from build123d import *

# Parameters (mm, degrees)
ESQUISSE2_R                = 7
ESQUISSE2_R_2              = 4
ESQUISSE2_R_3              = 23
BASE_EXTRUSION_DEPTH       = 2.5
ESQUISSE9_R                = 1.7
ENL_V_MAT_EXTRU_2_DEPTH    = 146.323213238
R_P_TITION_LIN_AIRE1_COUNT = 2
R_P_TITION_LIN_AIRE1_PITCH = 10
ESQUISSE10_R               = 1.7
ENL_V_MAT_EXTRU_3_DEPTH    = 146.323213238
R_P_TITION_LIN_AIRE2_COUNT = 2
R_P_TITION_LIN_AIRE2_PITCH = 83.5


with BuildPart() as part:
    # Esquisse2 → Base-Extrusion (new body)
    with BuildSketch(Plane.XY):
        with BuildLine():
            Line((-60.587831126, 50.043046358), (101.412168874, 50.043046358))
            ThreePointArc((101.412168874, 50.043046358), (136.412168874, 15.043046358), (101.412168874, -19.956953642))
            Line((101.412168874, -19.956953642), (-60.587831126, -19.956953642))
            ThreePointArc((-60.587831126, -19.956953642), (-95.587831126, 15.043046358), (-60.587831126, 50.043046358))
        make_face()
        with Locations((-60.587831126, 15.043046358)):
            Circle(ESQUISSE2_R, mode=Mode.SUBTRACT)
        with Locations((101.412168874, 15.043046358)):
            Circle(ESQUISSE2_R_2, mode=Mode.SUBTRACT)
        with Locations((51.412168874, 15.043046358)):
            Circle(ESQUISSE2_R_3, mode=Mode.SUBTRACT)
        with Locations((-10.587831126, 15.043046358)):
            Circle(ESQUISSE2_R_3, mode=Mode.SUBTRACT)
    extrude(amount=BASE_EXTRUSION_DEPTH)

    # Esquisse9 → Enlèv. mat.-Extru.2 (cut, through all)
    with BuildSketch(Plane.XY.offset(2.5)):
        with Locations((12.412168874, 37.043046358)):
            Circle(ESQUISSE9_R)
    enl_v_mat_extru_2 = extrude(amount=-ENL_V_MAT_EXTRU_2_DEPTH, mode=Mode.SUBTRACT)

    # Répétition linéaire1: Enlèv. mat.-Extru.2 ×2
    with Locations(*[(i * R_P_TITION_LIN_AIRE1_PITCH, 0, 0) for i in range(1, R_P_TITION_LIN_AIRE1_COUNT)]):
        add(enl_v_mat_extru_2, mode=Mode.SUBTRACT)

    # Esquisse10 → Enlèv. mat.-Extru.3 (cut, through all)
    with BuildSketch(Plane.XY.offset(2.5)):
        with Locations((-27.087831126, -13.956953642)):
            Circle(ESQUISSE10_R)
    enl_v_mat_extru_3 = extrude(amount=-ENL_V_MAT_EXTRU_3_DEPTH, mode=Mode.SUBTRACT)

    # Répétition linéaire2: Enlèv. mat.-Extru.3 ×2
    with Locations(*[(i * R_P_TITION_LIN_AIRE2_PITCH, 0, 0) for i in range(1, R_P_TITION_LIN_AIRE2_COUNT)]):
        add(enl_v_mat_extru_3, mode=Mode.SUBTRACT)


solid = part.part
Check sheet for the modelled part. Datum: model origin and axes. Units: mm. Round coordinates to 2 decimals unless told otherwise and drop trailing zeros. Loops run counter-clockwise (first coordinate to the right, second up) from the corner with the lowest first, then second, coordinate; pieces in that order, holes last. Notation, with made-up numbers: M 52,-2.75 L 71,-2.75 A24 cw 71,26.25 Z; hole C -7.75,47 d3. An arc over 180 degrees is marked long. One line per question, with ' | ' between items. Start each with the question number.
Item 1: Section check D-D (x = 35.5). Record the boundary of the cut face in (y, z), and give its area (3 significant figures).
Item 2: Section check C-C (z = 1.1). State how many separate pieces and enclosed holes the cut face has, and give its area (3 significant figures).
Item 3: Scan lines: probe 1 along X at (y, z) = (14, 0.85); probe 2 along X at (y, z) = (14.5, 1.05); probe 3 along Y at (x, z) = (51, 0.15). Record each from-to range of solid material in increasing order.
Item 4: Gauge pin test, flat ends, axial feed: pin 1 Ø5.5 at (x, y) = (56.41, -13.96) entering from -Z; pin 2 Ø7 at (x, y) = (101.41, 15.04) entering from +Z. Record the tip position at first contact, or that the pin passes through.
Item 5: Section check B-B (y = -6). Record the boundary of the cut face in (x, z), and give its area (3 significant figures).
Item 6: Section check A-A (x = 3.5). Record the boundary of the cut face in (y, z), and give its area (3 significant figures).
Item 7: Release check for a two-part mould opening along Y. For faces 1 (the face through (22, 16, 0)), 2 (the face through (-28.84, 1.05, 1.23)), 3 (the face through (136.404, 15.813, 1.232)), 4 (the face through (-65.75, 19.77, 1.23)) record: released by +Y, released by -Y, zero draft, split by the parting line, or undercut.
Worked out:
1) outline: M -19.96,0 L -1.56,0 L -1.56,2.5 L -19.96,2.5 Z; M 31.65,0 L 50.04,0 L 50.04,2.5 L 31.65,2.5 Z | area: 92.0 mm^2
2) separate pieces: 1 | enclosed holes: 8 | area: 11,600 mm^2
3) probe 1: -95.57 to -67.51, -53.67 to -33.56, 12.39 to 28.44, 74.39 to 97.55, 105.27 to 136.4 | probe 2: -95.58 to -67.57, -53.61 to -33.58, 12.41 to 28.42, 74.41 to 97.45, 105.38 to 136.41 | probe 3: -19.96 to -7.95, 38.04 to 50.04
4) pin 1: z = 0 | pin 2: through
5) outline: M -88.56,0 L -19.87,0 L -19.87,2.5 L -88.56,2.5 Z; M -1.3,0 L 42.13,0 L 42.13,2.5 L -1.3,2.5 Z; M 60.7,0 L 129.38,0 L 129.38,2.5 L 60.7,2.5 Z | area: 452 mm^2
6) outline: M -19.96,0 L -3.14,0 L -3.14,2.5 L -19.96,2.5 Z; M 33.22,0 L 50.04,0 L 50.04,2.5 L 33.22,2.5 Z | area: 84.1 mm^2
7) face 1: zero draft | face 2: undercut | face 3: split by the parting line | face 4: undercut
